```python
from build123d import *

# Parameters (mm, degrees)
SKETCH1_R           = 1.275
BOSS_EXTRUDE1_DEPTH = 6.5
SKETCH2_W           = 3.53
SKETCH2_H           = 1.96
BOSS_EXTRUDE2_DEPTH = 1.45
FILLET1_R           = 0.7
SKETCH3_W           = 3.2
SKETCH3_H           = 0.56
SKETCH3_H_2         = 0.5
BOSS_EXTRUDE3_DEPTH = 0.9
SKETCH4_W           = 1.2
SKETCH4_H           = 0.56
SKETCH4_H_2         = 0.5
BOSS_EXTRUDE4_DEPTH = 3.47
FILLET2_R           = 0.59
EXTRUDE_START       = -1.5
EXTRUDE_1_DEPTH     = 4
FILLET_1_R          = 0.5


with BuildPart() as part:
    # Sketch1 → Boss-Extrude1 (new body)
    with BuildSketch(Plane(origin=(0, 0, 0), x_dir=(0, 0, -1), z_dir=(1, 0, 0))):
        with BuildLine():
            Line((-37.373122581, 0), (-34.673122581, 0))
            Line((-34.673122581, 0), (-34.673122581, -0.45))
            Line((-34.673122581, -0.45), (-30.873122581, -0.45))
            Line((-30.873122581, -0.45), (-30.873122581, 0))
            Line((-30.873122581, 0), (-24.973122581, 0))
            Line((-24.973122581, 0), (-24.973122581, -0.45))
            Line((-24.973122581, -0.45), (-21.173122581, -0.45))
            Line((-21.173122581, -0.45), (-21.173122581, 0))
            Line((-21.173122581, 0), (-18.673122581, 0))
            ThreePointArc((-18.673122581, 0), (-18.31956919, 0.146446609), (-18.173122581, 0.5))
            Line((-18.173122581, 0.5), (-18.173122581, 9.02))
            ThreePointArc((-18.173122581, 9.02), (-18.31956919, 9.373553391), (-18.673122581, 9.52))
            Line((-18.673122581, 9.52), (-28.173122581, 9.52))
            Line((-28.173122581, 9.52), (-28.173122581, 10.16))
            Line((-28.173122581, 10.16), (-37.373122581, 10.16))
            ThreePointArc((-37.373122581, 10.16), (-37.726675972, 10.013553391), (-37.873122581, 9.66))
            Line((-37.873122581, 9.66), (-37.873122581, 0.5))
            ThreePointArc((-37.873122581, 0.5), (-37.726675972, 0.146446609), (-37.373122581, 0))
        make_face()
        with Locations((-32.773122581, 2.525)):
            Circle(SKETCH1_R, mode=Mode.SUBTRACT)
        with Locations((-23.073122581, 2.525)):
            Circle(SKETCH1_R, mode=Mode.SUBTRACT)
    extrude(amount=BOSS_EXTRUDE1_DEPTH)

    # Sketch2 → Boss-Extrude2 (add)
    with BuildSketch(Plane(origin=(0, 10.16, 0), x_dir=(1, 0, 0), z_dir=(0, 1, 0))):
        with Locations((3.635, -30.693122581)):
            Rectangle(SKETCH2_W, SKETCH2_H)
    extrude(amount=BOSS_EXTRUDE2_DEPTH)

    # Fillet1
    fillet1_edges = [part.edges().sort_by_distance(p)[0] for p in [
        (3.635, 11.61, 31.673122581),
        (3.635, 11.61, 29.713122581),
    ]]
    fillet(fillet1_edges, radius=FILLET1_R)

    # Sketch3 → Boss-Extrude3 (add)
    with BuildSketch(Plane(origin=(0, 0, 0), x_dir=(-1, 0, 0), z_dir=(0, -1, 0))):
        with Locations((-3.25, -36.193122581)):
            Rectangle(SKETCH3_W, SKETCH3_H)
        with Locations((-3.25, -27.223122581)):
            Rectangle(SKETCH3_W, SKETCH3_H_2)
        with Locations((-3.25, -20.023122581)):
            Rectangle(SKETCH3_W, SKETCH3_H_2)
    extrude(amount=BOSS_EXTRUDE3_DEPTH)

    # Sketch4 → Boss-Extrude4 (add)
    with BuildSketch(Plane(origin=(0, -0.9, 0), x_dir=(-1, 0, 0), z_dir=(0, -1, 0))):
        with Locations((-3.25, -36.193122581)):
            Rectangle(SKETCH4_W, SKETCH4_H)
        with Locations((-3.25, -27.223122581)):
            Rectangle(SKETCH4_W, SKETCH4_H_2)
        with Locations((-3.25, -20.023122581)):
            Rectangle(SKETCH4_W, SKETCH4_H_2)
    extrude(amount=BOSS_EXTRUDE4_DEPTH)

    # Fillet2
    fillet2_edges = [part.edges().sort_by_distance(p)[0] for p in [
        (2.65, -4.37, 36.193122581),
        (3.85, -4.37, 36.193122581),
        (2.65, -4.37, 27.223122581),
        (3.85, -4.37, 27.223122581),
        (3.85, -4.37, 20.023122581),
        (2.65, -4.37, 20.023122581),
    ]]
    fillet(fillet2_edges, radius=FILLET2_R)

    # Эскиз1 → Бобышка-Вытянуть1 (add)
    with BuildSketch(Plane(origin=(6.5, 0, 0), x_dir=(0, 0, -1), z_dir=(1, 0, 0)).offset(EXTRUDE_START)):
        with BuildLine():
            Line((-35.033122581, 10.16), (-34.820611294, 10.16))
            Line((-34.820611294, 10.16), (-34.820611294, 11.065475419))
            Line((-34.820611294, 11.065475419), (-16.983122581, 13.639958326))
            Line((-16.983122581, 13.639958326), (-17.327590515, 16.026629013))
            ThreePointArc((-17.327590515, 16.026629013), (-19.152479599, 14.674662016), (-21.2856409, 15.454186098))
            Line((-21.2856409, 15.454186098), (-20.970513986, 13.279774136))
            Line((-20.970513986, 13.279774136), (-35.033122581, 11.241748905))
            Line((-35.033122581, 11.241748905), (-35.033122581, 10.16))
        make_face()
        with BuildLine():
            ThreePointArc((-21.2856409, 15.454186098), (-19.152479599, 14.674662016), (-17.327590515, 16.026629013))
            Line((-17.327590515, 16.026629013), (-17.515806862, 17.330699412))
            ThreePointArc((-17.515806862, 17.330699412), (-19.781572094, 19.024405415), (-21.474617523, 16.75814654))
            Line((-21.474617523, 16.75814654), (-21.2856409, 15.454186098))
        make_face()
        with BuildLine():
            Line((-17.515806862, 17.330699412), (-17.327590515, 16.026629013))
            ThreePointArc((-17.327590515, 16.026629013), (-17.157809946, 16.523285896), (-17.100295646, 17.045))
            ThreePointArc((-17.100295646, 17.045), (-17.801774905, 18.738520741), (-19.495295646, 19.44))
            ThreePointArc((-19.495295646, 19.44), (-21.680018087, 18.026332182), (-21.2856409, 15.454186098))
            Line((-21.2856409, 15.454186098), (-21.474617523, 16.75814654))
            ThreePointArc((-21.474617523, 16.75814654), (-19.781572094, 19.024405415), (-17.515806862, 17.330699412))
        make_face()
    extrude(amount=-EXTRUDE_1_DEPTH)

    # Скругление1
    fillet_1_edges = [part.edges().sort_by_distance(p)[0] for p in [
        (3, 11.065475419, 34.820611294),
        (3, 11.241748905, 35.033122581),
    ]]
    fillet(fillet_1_edges, radius=FILLET_1_R)


solid = part.part
```
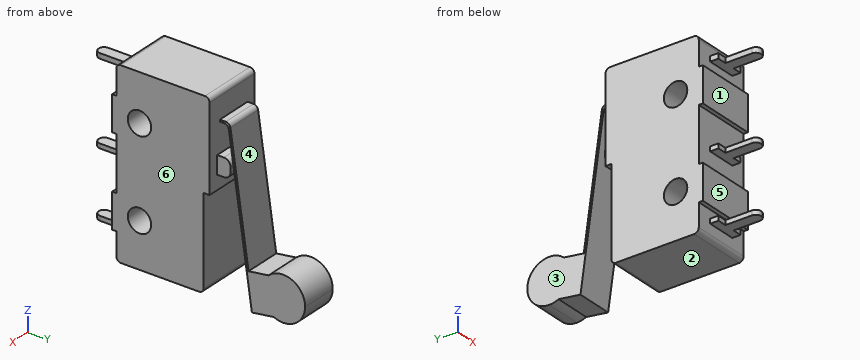
CAD build for the part. Positions are in the model's coordinates, mm. Face numbers are marked on the shaded views. A direction names the side the tool comes from. Coordinates: 2 decimals unless noted, no trailing zeros. Loops run counter-clockwise (first coordinate to the right, second up) from the corner with the lowest first, then second, coordinate; pieces in that order, holes last. Notation, with made-up numbers: (59, 39) - (111, 39) arc R19 ccw to (111, 63) - close; hole circle Ø11 at (7, -18). An arc over 180 degrees is marked (long way). Return JSON: item names as keys, results as strings.
1. Band-saw the part on C-C (z = 26). Give the cut face in (x, y).
Result:
{"outline": "(0, 0) - (6.5, 0) - (6.5, 9.52) - (0, 9.52) - close; (1, 12.34) - (5, 12.34) - (5, 12.55) - (1, 12.55) - close"}
2. Band-saw the part on A-A (z = 28.5). Give the cut face in (x, y).
Result:
{"outline": "(0, 0) - (6.5, 0) - (6.5, 10.16) - (0, 10.16) - close; (1, 11.98) - (5, 11.98) - (5, 12.19) - (1, 12.19) - close"}
3. Band-saw the part on D-D (z = 36.75). Give the cut face in (x, y), and give its area (3 significant figures).
Result:
{"outline": "(0, 0) - (6.5, 0) - (6.5, 10.16) - (0, 10.16) - close", "area": "66.0 mm2"}
4. Probe L1, parallel to Z at x = 2.25, y = 10.5; L2, parallel to Y at x = 3.75, z = 24; L3, parallel to X at y = 16.75, z = 19.5. List the from-to ranges inside material, lowest first. Write a range as from..to.
Result:
{"L1": "z = 29.71..31.67, 34.82..35.03", "L2": "y = -0.45..1.65, 3.4..9.52, 12.63..12.84", "L3": "x = 1..5"}
5. Drop flat-ended pins along their axis: pin 1 (0.6 mm diameter, centred on y = -0.5, z = 27, fed in from +X); pin 2 (2 mm diameter, centred on x = 3.5, z = 34.5, fed in from +Y); pin 3 (1 mm diameter, centred on x = 3, y = -2, fed in from +Z); pin 4 (12 mm diameter, centred on y = 6.5, z = 25.5, fed in from -X). Give the stop position or say it passes through.
Result:
{"pin 1": "stops at x = 4.85", "pin 2": "stops at y = 11.46", "pin 3": "stops at z = 36.47", "pin 4": "stops at x = 0"}
6. 3-axis set-ups, long thin cutter, end or side, ignore diameter. For the marked faces 1, 2 and 3: which of +Z, -Z, +X, -X, +Y, -Y reach the whole face in a straight line?
Result:
{"face 1": "+X, -X, -Y", "face 2": "-Z, +X, -X, -Y", "face 3": "+Z, -Z, -X, +Y"}
7. Mould opens along Z. For the marked faces 4, 5 and 6 say: released by +Z, released by -Z, zero draft, split by the parting line, or undercut.
Result:
{"face 4": "released by +Z", "face 5": "undercut", "face 6": "zero draft"}
8. Band-saw the part on B-B (y = 4.5). Give the cut face in (x, z), and give its area (3 significant figures).
Result:
{"outline": "(0, 18.17) - (6.5, 18.17) - (6.5, 37.87) - (0, 37.87) - close", "area": "128 mm2"}
